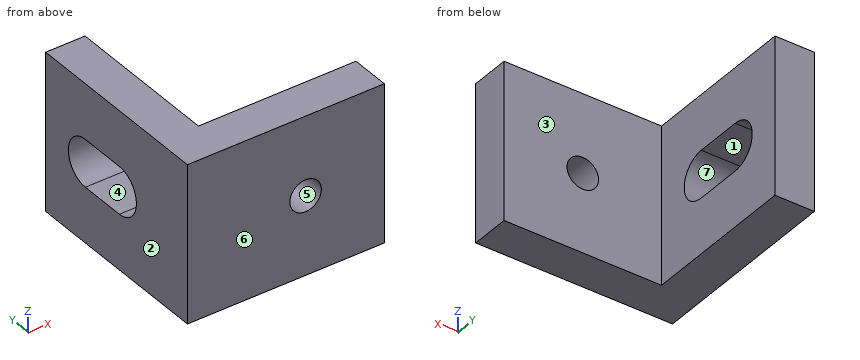
```python
from build123d import *

# Parameters (mm, degrees)
SKETCH1_W           = 20
SKETCH1_H           = 20
SKETCH1_R           = 2
BOSS_EXTRUDE1_DEPTH = 5
SKETCH2_W           = 5
SKETCH2_H           = 20
BOSS_EXTRUDE2_DEPTH = 25
SKETCH3_W           = 6
SKETCH3_H           = 6
CUT_EXTRUDE1_DEPTH  = 25


with BuildPart() as part:
    # Sketch1 → Boss-Extrude1 (new body)
    with BuildSketch(Plane(origin=(0, 0, 0), x_dir=(1, 0, 0), z_dir=(0, 1, 0))):
        Rectangle(SKETCH1_W, SKETCH1_H)
        Circle(SKETCH1_R, mode=Mode.SUBTRACT)
    extrude(amount=BOSS_EXTRUDE1_DEPTH)

    # Sketch2 → Boss-Extrude2 (add)
    with BuildSketch(Plane.XZ):
        with Locations((-12.5, 0)):
            Rectangle(SKETCH2_W, SKETCH2_H)
    extrude(amount=-BOSS_EXTRUDE2_DEPTH)

    # Sketch3 → Cut-Extrude1 (cut)
    with BuildSketch(Plane(origin=(-10, 0, 0), x_dir=(0, 0, -1), z_dir=(1, 0, 0))):
        with BuildLine():
            ThreePointArc((-3, 18), (0, 21), (3, 18))
            Line((3, 18), (-3, 18))
        make_face()
        with Locations((0, 15)):
            Rectangle(SKETCH3_W, SKETCH3_H)
        with BuildLine():
            ThreePointArc((3, 12), (0, 9), (-3, 12))
            Line((-3, 12), (3, 12))
        make_face()
    extrude(amount=-CUT_EXTRUDE1_DEPTH, mode=Mode.SUBTRACT)


solid = part.part
```
Design review of the part built by this model. Coordinates are the model's own, in mm. Face numbers are marked on the shaded views. A direction names the side the tool comes from. Give positions to 0.01 mm unless a question says otherwise; leave off trailing zeros. Write each loop counter-clockwise with the first axis right and the second up, starting at its lowest first coordinate (ties: lowest second). Pieces come first, ordered by that corner, then holes.
(1) Add section D-D (x = -13.5). Give the boundary of the cut face in (y, z).
Checked values:
outline: (0, -10) - (25, -10) - (25, 10) - (0, 10) - close; hole (12, -3) - (18, -3) arc R3 ccw to (18, 3) - (12, 3) arc R3 ccw to start
(2) Add section A-A (y = 13.5). Give the boundary of the cut face in (x, z).
Checked values:
outline: (-15, -10) - (-10, -10) - (-10, -3) - (-15, -3) - close; (-15, 3) - (-10, 3) - (-10, 10) - (-15, 10) - close
(3) Wall thickness on line 1 along Z through (x, y) = (0, 1.9); line 2 along X through (y, z) = (2.3, 0); line 3 along Y through (x, z) = (-9.5, -2.25): over which ranges is each line inside the solid? List them lowest first.
Checked values:
line 1: z = -10 to -2, 2 to 10
line 2: x = -15 to -2, 2 to 10
line 3: y = 0 to 5
(4) Clearance check with flat-ended pins moving along their axes: pin 1 Ø10 at (x, z) = (0, -2.5) entering from +Y; pin 2 Ø1.5 at (y, z) = (19.5, -1) entering from +X. State where each tip first meets the part, or that it passes through.
Checked values:
pin 1: stops at y = 5
pin 2: passes through
(5) Mouldability with a two-part tool opening along Y and no side actions: class the marked faces 4, 5, 6 and 7 as +Y half, -Y half, draft (parallel to the pull), parting line (faces both ways), or undercut.
Checked values:
face 4: undercut
face 5: draft
face 6: -Y half
face 7: undercut
(6) Add section C-C (z = 0). Give the boundary of the cut face in (x, y).
Checked values:
outline: (-15, 0) - (-2, 0) - (-2, 5) - (-10, 5) - (-10, 9) - (-15, 9) - close; (-15, 21) - (-10, 21) - (-10, 25) - (-15, 25) - close; (2, 0) - (10, 0) - (10, 5) - (2, 5) - close
(7) Tool access review of the marked faces 1, 2 and 3: name each direction out of +Z, -Z, +X, -X, +Y, -Y from which nothing blocks a thin tool from reaching the whole face with its end or side.
Checked values:
face 1: +X, -X
face 2: +Z, -Z, -X, +Y, -Y
face 3: +Z, -Z, +X, +Y
(8) Add section B-B (x = 0). Give the boundary of the cut face in (y, z).
Checked values:
outline: (0, -10) - (5, -10) - (5, -2) - (0, -2) - close; (0, 2) - (5, 2) - (5, 10) - (0, 10) - close
